from build123d import *

# Parameters (mm, degrees)
CROQUIS1_W              = 508
CROQUIS1_H              = 38.1
SALIENTE_EXTRUIR1_DEPTH = 38.1
CROQUIS2_R              = 6.35
SALIENTE_EXTRUIR2_DEPTH = 12.7
CROQUIS3_R              = 6.35
SALIENTE_EXTRUIR3_DEPTH = 12.7
CROQUIS4_R              = 6.35
CORTAR_EXTRUIR1_DEPTH   = 12.7


with BuildPart() as part:
    # Croquis1 → Saliente-Extruir1 (new body)
    with BuildSketch(Plane(origin=(0, 0, 0), x_dir=(1, 0, 0), z_dir=(0, 1, 0))):
        Rectangle(CROQUIS1_W, CROQUIS1_H)
    extrude(amount=SALIENTE_EXTRUIR1_DEPTH)

    # Croquis2 → Saliente-Extruir2 (add)
    with BuildSketch(Plane.ZY.offset(254)):
        with Locations((0, 19.05)):
            Circle(CROQUIS2_R)
    extrude(amount=SALIENTE_EXTRUIR2_DEPTH)

    # Croquis3 → Saliente-Extruir3 (add)
    with BuildSketch(Plane(origin=(254, 0, 0), x_dir=(0, 0, -1), z_dir=(1, 0, 0))):
        with Locations((0, 19.05)):
            Circle(CROQUIS3_R)
    extrude(amount=SALIENTE_EXTRUIR3_DEPTH)

    # Croquis4 → Cortar-Extruir1 (cut)
    with BuildSketch(Plane(origin=(0, 38.1, 0), x_dir=(1, 0, 0), z_dir=(0, 1, 0))):
        Circle(CROQUIS4_R)
    extrude(amount=-CORTAR_EXTRUIR1_DEPTH, mode=Mode.SUBTRACT)


solid = part.part
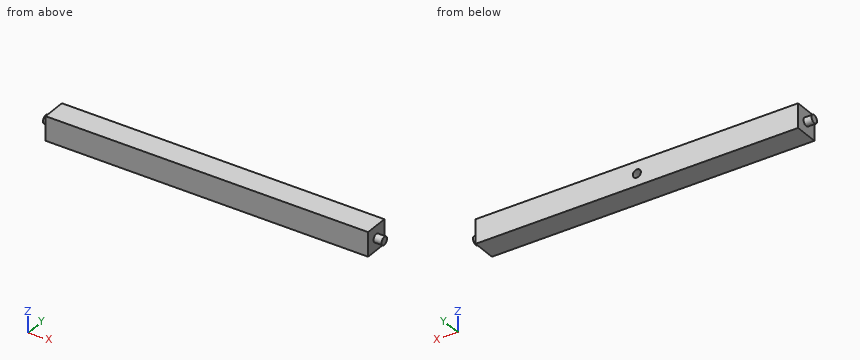
Model file for the job. Use its own axes, mm. Round coordinates to 2 decimals unless told otherwise and drop trailing zeros. Loops run counter-clockwise (first coordinate to the right, second up) from the corner with the lowest first, then second, coordinate; pieces in that order, holes last.
1. Wall check: probe 1 along Z at (x, y) = (0, 28); probe 2 along X at (y, z) = (31, 0); probe 3 along X at (y, z) = (14, 12). Give the ranges that are in metal, low to high.
Check values:
probe 1: z = -19.05 to -6.35, 6.35 to 19.05
probe 2: x = -254 to -6.35, 6.35 to 254
probe 3: x = -254 to 254
2. Drop flat-ended pins along their axis: P1, Ø2, axis at x = 196.5, z = -3, coming from the -Y side; P2, Ø1, axis at y = 9.5, z = 0.5, coming from the +X side; P3, Ø1, axis at y = 25.5, z = -11.5, coming from the -X side. Give the stop position or say it passes through.
Check values:
P1: stops at y = 0
P2: stops at x = 254
P3: stops at x = -254
3. Band-saw the part on C-C, the plane x = 0. List the corners of the cut face in (y, z), and give its area (3 significant figures).
Check values:
outline: (0, -19.05) - (38.1, -19.05) - (38.1, -6.35) - (25.4, -6.35) - (25.4, 6.35) - (38.1, 6.35) - (38.1, 19.05) - (0, 19.05) - close
area: 1,290 mm2
4. Band-saw the part on B-B, the plane z = 0. List the corners of the cut face in (x, y).
Check values:
outline: (-266.7, 12.7) - (-254, 12.7) - (-254, 0) - (254, 0) - (254, 12.7) - (266.7, 12.7) - (266.7, 25.4) - (254, 25.4) - (254, 38.1) - (6.35, 38.1) - (6.35, 25.4) - (-6.35, 25.4) - (-6.35, 38.1) - (-254, 38.1) - (-254, 25.4) - (-266.7, 25.4) - close
5. Band-saw the part on A-A, the plane y = 19.05. List the corners of the cut face in (x, z), and give its area (3 significant figures).
Check values:
outline: (-266.7, -6.35) - (-254, -6.35) - (-254, -19.05) - (254, -19.05) - (254, -6.35) - (266.7, -6.35) - (266.7, 6.35) - (254, 6.35) - (254, 19.05) - (-254, 19.05) - (-254, 6.35) - (-266.7, 6.35) - close
area: 19,700 mm2
